Build history of the part. All positions in model axes, mm. A direction names the side the tool comes from. Round coordinates to 2 decimals unless told otherwise and drop trailing zeros. Write each loop counter-clockwise with the first axis right and the second up, starting at its lowest first coordinate (ties: lowest second). Pieces come first, ordered by that corner, then holes. Notation, with made-up numbers: M -23.5,-22 L -18.5,-22 A24 cw -18.5,-6 Z; hole C 28.25,53.25 d2. An arc over 180 degrees is marked long. Use a Markdown table: item, result.
from build123d import *

# Parameters (mm, degrees)
SKETCH1_W                = 26.611
SKETCH1_H                = 70
SKETCH1_R                = 3
BOSS_EXTRUDE1_DEPTH      = 4.5
BOSS_EXTRUDE1_2_DEPTH    = 4.5
SKETCH2_W                = 61.722
SKETCH2_H                = 70
SKETCH2_R                = 5.5
BOSS_EXTRUDE2_DEPTH      = 4.5
SKETCH3_W                = 3
SKETCH3_H                = 70
BOSS_EXTRUDE3_DEPTH      = 5
CHAMFER1_SIZE            = 5
CUT_EXTRUDE1_DEPTH       = 53.134549552
CUT_EXTRUDE1_DEPTH_BACK  = 53.134549552
SKETCH4_W                = 20.5
SKETCH4_H                = 10.5
MIRROR1_OUTLINE_R        = 5.5
MIRROR1_DEPTH            = 9
MIRROR1_START            = 4.5
MIRROR1_2_OUTLINE_W      = 8.5
MIRROR1_2_OUTLINE_H      = 59.5
MIRROR1_2_DEPTH          = 4.5
MIRROR1_3_OUTLINE_R      = 5.5
MIRROR1_3_OUTLINE_R_2    = 3
MIRROR1_3_DEPTH          = 4.5
MIRROR1_START_2          = -111.044
MIRROR1_4_DEPTH          = 70
SKETCH5_R                = 1.25
BOSS_EXTRUDE4_DEPTH      = 30
SKETCH6_W                = 1.1
SKETCH6_H                = 59.5
BOSS_EXTRUDE5_DEPTH      = 5
SKETCH7_W                = 6
SKETCH7_H                = 4
CUT_EXTRUDE2_DEPTH       = 2
CHAMFER2_SIZE            = 2
CHAMFER3_SIZE            = 2
CHAMFER2_OF_MIRROR2_SIZE = 2
CHAMFER3_OF_MIRROR2_SIZE = 2


with BuildPart() as part:
    # Sketch1 → Boss-Extrude1 (new body)
    with BuildSketch(Plane.XY):
        with Locations((17.5555, -6.044)):
            Rectangle(SKETCH1_W, SKETCH1_H)
        with Locations((24.8412, 19.05)):
            Circle(SKETCH1_R, mode=Mode.SUBTRACT)
        with Locations((24.8412, -19.05)):
            Circle(SKETCH1_R, mode=Mode.SUBTRACT)
    extrude(amount=BOSS_EXTRUDE1_DEPTH)



with BuildPart() as body_2:
    # Sketch1 → Boss-Extrude1 2 (new body)
    with BuildSketch(Plane.XY):
        with Locations((-17.5555, -6.044)):
            Rectangle(SKETCH1_W, SKETCH1_H)
        with Locations((-24.8158, -19.05)):
            Circle(SKETCH1_R, mode=Mode.SUBTRACT)
        with Locations((-24.8158, 19.05)):
            Circle(SKETCH1_R, mode=Mode.SUBTRACT)
    extrude(amount=BOSS_EXTRUDE1_2_DEPTH)


with BuildPart() as part_1:
    add(part.part)

    add(body_2.part)  # Boss-Extrude2 merges body 2
    # Sketch2 → Boss-Extrude2 (add)
    with BuildSketch(Plane.XY.offset(4.5)):
        with Locations((0, -6.044)):
            Rectangle(SKETCH2_W, SKETCH2_H)
        with Locations((24.8412, -19.05)):
            Circle(SKETCH2_R, mode=Mode.SUBTRACT)
        with Locations((-24.8158, -19.05)):
            Circle(SKETCH2_R, mode=Mode.SUBTRACT)
        with Locations((-24.8158, 19.05)):
            Circle(SKETCH2_R, mode=Mode.SUBTRACT)
        with Locations((24.8412, 19.05)):
            Circle(SKETCH2_R, mode=Mode.SUBTRACT)
    extrude(amount=BOSS_EXTRUDE2_DEPTH)

    # Sketch3 → Boss-Extrude3 (add)
    with BuildSketch(Plane.XY.offset(9)):
        with Locations((11.75, -6.044)):
            Rectangle(SKETCH3_W, SKETCH3_H)
        with Locations((-11.75, -6.044)):
            Rectangle(SKETCH3_W, SKETCH3_H)
    extrude(amount=BOSS_EXTRUDE3_DEPTH)

    # Chamfer1
    chamfer1_edges = [part_1.edges().sort_by_distance(p)[0] for p in [
        (-13.25, -6.044, 9),
        (13.25, -6.044, 9),
    ]]
    chamfer(chamfer1_edges, length=CHAMFER1_SIZE - 0.0001)  # a hair under: the kernel refuses the full size

    # Sketch4 → Cut-Extrude1 (cut, two sides: drawn at the far end of the back side and taken through both)
    with BuildSketch(Plane.XY.offset(9).offset(-CUT_EXTRUDE1_DEPTH_BACK)):
        with Locations((0, -35.794)):
            Rectangle(SKETCH4_W, SKETCH4_H)
        with BuildLine():
            Line((-2.5, -23.544), (-2.5, -19.544))
            ThreePointArc((-2.5, -19.544), (0, -17.044), (2.5, -19.544))
            Line((2.5, -19.544), (2.5, -23.544))
            ThreePointArc((2.5, -23.544), (0, -26.044), (-2.5, -23.544))
        make_face()
    extrude(amount=CUT_EXTRUDE1_DEPTH + CUT_EXTRUDE1_DEPTH_BACK, mode=Mode.SUBTRACT)

    # Mirror1: read off the stored shape, not the designer's step
    # Mirror1 outline → Mirror1 (add)
    # profile 1 of 2: a face of its own
    with BuildSketch(Plane.XY):
        Polygon((30.861, -111.044), (30.861, -41.044), (10.25, -41.044), (10.25, -51.544), (4.25, -51.544), (4.25, -111.044), align=None)
        with Locations((24.8412, -101.138)):
            Circle(MIRROR1_OUTLINE_R, mode=Mode.SUBTRACT)
        with Locations((24.8412, -63.038)):
            Circle(MIRROR1_OUTLINE_R, mode=Mode.SUBTRACT)
    # profile 2 of 2: a face of its own
    with BuildSketch(Plane.XY):
        Polygon((-4.25, -111.044), (-4.25, -51.544), (-10.25, -51.544), (-10.25, -41.044), (-30.861, -41.044), (-30.861, -111.044), align=None)
        with Locations((-24.8158, -63.038)):
            Circle(MIRROR1_OUTLINE_R, mode=Mode.SUBTRACT)
        with Locations((-24.8158, -101.138)):
            Circle(MIRROR1_OUTLINE_R, mode=Mode.SUBTRACT)
    extrude(amount=MIRROR1_DEPTH)

    # Mirror1 2 outline → Mirror1 2 (add)
    with BuildSketch(Plane.XY.offset(MIRROR1_START)):
        with Locations((0, -81.294)):
            Rectangle(MIRROR1_2_OUTLINE_W, MIRROR1_2_OUTLINE_H)
        with BuildLine():
            Line((-2.5, -62.544), (-2.5, -58.544))
            ThreePointArc((-2.5, -58.544), (0, -56.044), (2.5, -58.544))
            Line((2.5, -58.544), (2.5, -62.544))
            ThreePointArc((2.5, -62.544), (0, -65.044), (-2.5, -62.544))
        make_face(mode=Mode.SUBTRACT)
    extrude(amount=MIRROR1_2_DEPTH)

    # Mirror1 3 outline → Mirror1 3 (add)
    # profile 1 of 4: a face of its own
    with BuildSketch(Plane.XY):
        with Locations((24.8412, -63.038)):
            Circle(MIRROR1_3_OUTLINE_R)
        with Locations((24.8412, -63.038)):
            Circle(MIRROR1_3_OUTLINE_R_2, mode=Mode.SUBTRACT)
    # profile 2 of 4: a face of its own
    with BuildSketch(Plane.XY):
        with Locations((-24.8158, -63.038)):
            Circle(MIRROR1_3_OUTLINE_R)
        with Locations((-24.8158, -63.038)):
            Circle(MIRROR1_3_OUTLINE_R_2, mode=Mode.SUBTRACT)
    # profile 3 of 4: a face of its own
    with BuildSketch(Plane.XY):
        with Locations((-24.8158, -101.138)):
            Circle(MIRROR1_3_OUTLINE_R)
        with Locations((-24.8158, -101.138)):
            Circle(MIRROR1_3_OUTLINE_R_2, mode=Mode.SUBTRACT)
    # profile 4 of 4: a face of its own
    with BuildSketch(Plane.XY):
        with Locations((24.8412, -101.138)):
            Circle(MIRROR1_3_OUTLINE_R)
        with Locations((24.8412, -101.138)):
            Circle(MIRROR1_3_OUTLINE_R_2, mode=Mode.SUBTRACT)
    extrude(amount=MIRROR1_3_DEPTH)

    # Mirror1 4 outline → Mirror1 4 (add)
    with BuildSketch(Plane(origin=(0, 0, 0), x_dir=(1, 0, 0), z_dir=(0, 1, 0)).offset(MIRROR1_START_2)):
        Polygon((-10.25, -14), (-10.25, -9), (-18.25, -9), (-13.25, -14), align=None)
        Polygon((10.25, -9), (10.25, -14), (13.25, -14), (18.25, -9), align=None)
    extrude(amount=MIRROR1_4_DEPTH)

    # Sketch5 → Boss-Extrude4 (add)
    with BuildSketch(Plane.XZ.offset(111.044)):
        with BuildLine():
            Line((-13.25, 14), (-13.25, 9))
            Line((-13.25, 9), (13.25, 9))
            Line((13.25, 9), (13.25, 14))
            ThreePointArc((13.25, 14), (0, 19.488329701), (-13.25, 14))
        make_face()
        with Locations(Location((0, 14, 0), (0, 0, 270))):
            Circle(SKETCH5_R, mode=Mode.SUBTRACT)
    extrude(amount=-BOSS_EXTRUDE4_DEPTH)

    # Sketch6 → Boss-Extrude5 (add)
    with BuildSketch(Plane.XY.offset(9)):
        with Locations((-9.7, -0.794)):
            Rectangle(SKETCH6_W, SKETCH6_H)
        with Locations((9.7, -0.794)):
            Rectangle(SKETCH6_W, SKETCH6_H)
    boss_extrude5 = extrude(amount=BOSS_EXTRUDE5_DEPTH)

    # Sketch7 → Cut-Extrude2 (cut)
    with BuildSketch(Plane.XY.offset(9)):
        with Locations((0, -14.544)):
            Rectangle(SKETCH7_W, SKETCH7_H)
        with Locations((0, -28.544)):
            Rectangle(SKETCH7_W, SKETCH7_H)
    cut_extrude2 = extrude(amount=-CUT_EXTRUDE2_DEPTH, mode=Mode.SUBTRACT)

    # Chamfer2
    chamfer2_edges = [part_1.edges().sort_by_distance(p)[0] for p in [
        (0, -26.544, 7),
    ]]
    chamfer(chamfer2_edges, length=CHAMFER2_SIZE - 0.0001)  # a hair under: the kernel refuses the full size

    # Chamfer3
    chamfer3_edges = [part_1.edges().sort_by_distance(p)[0] for p in [
        (0, -12.544, 7),
    ]]
    chamfer(chamfer3_edges, length=CHAMFER3_SIZE - 0.0001)  # a hair under: the kernel refuses the full size

    # Mirror2: Boss-Extrude5, Cut-Extrude2 across plane
    add(boss_extrude5.mirror(Plane(origin=(0, -41.044, 0), x_dir=(0, 0, 1), z_dir=(0, -1, 0))))
    add(cut_extrude2.mirror(Plane(origin=(0, -41.044, 0), x_dir=(0, 0, 1), z_dir=(0, -1, 0))), mode=Mode.SUBTRACT)

    # Chamfer2 of Mirror2
    chamfer2_of_mirror2_edges = [part_1.edges().sort_by_distance(p)[0] for p in [
        (0, -55.544, 7),
    ]]
    chamfer(chamfer2_of_mirror2_edges, length=CHAMFER2_OF_MIRROR2_SIZE - 0.0001)  # a hair under: the kernel refuses the full size

    # Chamfer3 of Mirror2
    chamfer3_of_mirror2_edges = [part_1.edges().sort_by_distance(p)[0] for p in [
        (0, -69.544, 7),
    ]]
    chamfer(chamfer3_of_mirror2_edges, length=CHAMFER3_OF_MIRROR2_SIZE - 0.0001)  # a hair under: the kernel refuses the full size


solid = part_1.part
Q1. Drill centre lines: L1, parallel to X at y = 10, z = 1; L2, parallel to Y at x = -27, z = 3.5; L3, parallel to Y at x = 9.5, z = 3. Where is each one in solid material? Low to high.
Response values:
| item | result |
|---|---|
| L1 | x = -30.86 to -4.25, 4.25 to 30.86 |
| L2 | y = -111.04 to -103.19, -99.08 to -65.09, -60.98 to -21.11, -16.99 to 16.99, 21.11 to 28.96 |
| L3 | y = -111.04 to -51.54, -30.54 to 28.96 |
Q2. Drop flat-ended pins along their axis: P1, Ø1.6, axis at x = -1, y = -15.5, coming from the +Z side; P2, Ø14.5, axis at x = -24.82, y = -101.14, coming from the +Z side; P3, Ø2.5, axis at y = 2.5, z = 12.5, coming from the -X side. Give the stop position or say it passes through.
Response values:
| item | result |
|---|---|
| P1 | stops at z = 7 |
| P2 | stops at z = 9.68 |
| P3 | stops at x = -16 |
Q3. Cut at B-B on y = -75.5. Give the cut face in (x, z).
Response values:
| item | result |
|---|---|
| outline | M -30.86,0 L -4.25,0 L -4.25,4.5 L 4.25,4.5 L 4.25,0 L 30.86,0 L 30.86,9 L 18.25,9 L 13.25,14 L 9.15,14 L 9.15,9 L -9.15,9 L -9.15,14 L -13.25,14 L -18.25,9 L -30.86,9 Z |
Q4. Two-plate mould, pull along X, no slides. Class faces 1 (the cylindrical face through (0.05, -96.25, 15.25)), 2 (the flat face through (-30.861, -42, 4)), 3 (the flat face through (17, -40, 0)): +X half, -X half, draft (parallel to the pull), parting line (faces both ways), or undercut.
Response values:
| item | result |
|---|---|
| face 1 | undercut |
| face 2 | -X half |
| face 3 | draft |
Q5. Cut at A-A on z = 2. Count the separate pieces of the cut face and the enclosed holes in it, and give its area (3 significant figures).
Response values:
| item | result |
|---|---|
| separate pieces | 2 |
| enclosed holes | 8 |
| area | 6,970 mm2 |
Q6. Which spindle directions (+Z, -Z, +X, -X, +Y, -Y) get a long thin tool onto all of the face, cutting with end or side? Do faces 4 (the flat face through (9.15, -1, 11)), 5 (the cylindrical face through (-29.18, 15.7, 6.72)), 6 (the cylindrical face through (0.055, -26.043, 6.718)), 7 (the flat face through (-4.25, -1, 2)), 8 (the flat face through (11, -27, 14)). Say none if no direction does.
Response values:
| item | result |
|---|---|
| face 4 | +Z, +Y |
| face 5 | +Z |
| face 6 | +Z, -Z |
| face 7 | -Z, +Y, -Y |
| face 8 | +Z, +X, -X, +Y |
